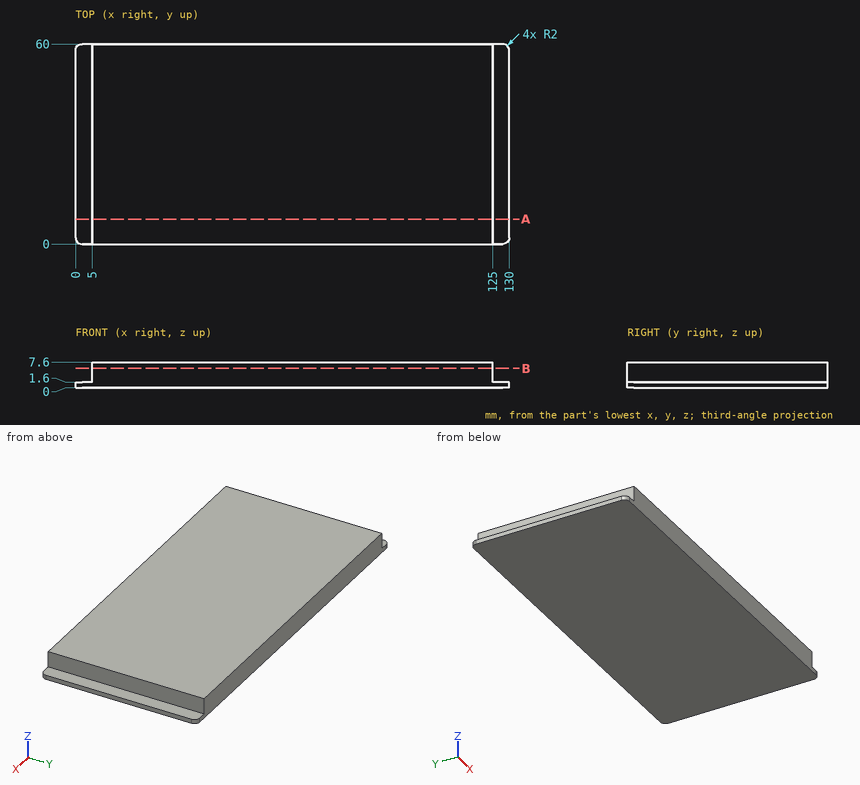
Verification items for this drawing (mm, ordinates from the low corner). Give positions to 0.01 mm unless a question says otherwise; leave off trailing zeros. Order: outer loops, then holes, each group sorted by start corner. A loop starts at its lowest first (then second) coordinate and runs counter-clockwise, first axis right, second up.
1) Gauge pin test, flat ends, axial feed: pin 1 (4 mm diameter, centred on y = 20.5, z = 5, fed in from +X); pin 2 (1.8 mm diameter, centred on y = 29.5, z = 4, fed in from -X); pin 3 (12 mm diameter, centred on x = 21, y = 24.5, fed in from -Z); pin 4 (5.5 mm diameter, centred on x = 128, y = 36, fed in from +Z). Record the tip position at first contact, or that the pin passes through.
Results are:
pin 1: stops at x = 125
pin 2: stops at x = 5
pin 3: stops at z = 0
pin 4: stops at z = 1.6
2) Cross-section at B-B (z = 5.75). Record the boundary of the cut face in (x, y).
Results are:
outline: (5, 0) - (125, 0) - (125, 60) - (5, 60) - close
3) Cross-section at A-A (y = 7.5). Record the boundary of the cut face in (x, z).
Results are:
outline: (0, 0) - (130, 0) - (130, 1.6) - (125, 1.6) - (125, 7.6) - (5, 7.6) - (5, 1.6) - (0, 1.6) - close
4) Material ranges on probe 1 along X at (y, z) = (56.5, 4), recorded low to high.
Results are:
probe 1: x = 5 to 125
